```python
from build123d import *

# Parameters (mm, degrees)
SKETCH1_W           = 38.1
SKETCH1_H           = 38.1
SKETCH1_R           = 1.27
BOSS_EXTRUDE1_DEPTH = 6.35
CUT_EXTRUDE1_DEPTH  = 5.08
CUT_EXTRUDE2_REACH  = 29.679
SKETCH3_W           = 9.398
SKETCH3_H           = 21.59
SKETCH4_W           = 2.320401775
SKETCH4_H           = 5.08
SKETCH4_R           = 3.101894328
CUT_EXTRUDE3_DEPTH  = 28.679008291


with BuildPart() as part:
    # Sketch1 → Boss-Extrude1 (new body)
    with BuildSketch(Plane(origin=(0, 0, 0), x_dir=(1, 0, 0), z_dir=(0, 1, 0))):
        Rectangle(SKETCH1_W, SKETCH1_H)
        with Locations(Location((-17.018, 17.018, 0), (0, 0, 270))):
            Circle(SKETCH1_R, mode=Mode.SUBTRACT)
        with Locations(Location((-17.018, -17.018, 0), (0, 0, 90))):
            Circle(SKETCH1_R, mode=Mode.SUBTRACT)
        with Locations(Location((17.018, -17.018, 0), (0, 0, 270))):
            Circle(SKETCH1_R, mode=Mode.SUBTRACT)
        with Locations(Location((17.018, 17.018, 0), (0, 0, 90))):
            Circle(SKETCH1_R, mode=Mode.SUBTRACT)
    extrude(amount=BOSS_EXTRUDE1_DEPTH)

    # Sketch2 → Cut-Extrude1 (cut)
    with BuildSketch(Plane(origin=(0, 6.35, 0), x_dir=(1, 0, 0), z_dir=(0, 1, 0))):
        with BuildLine():
            Line((18.256262039, 13.97), (18.256262039, -13.97))
            ThreePointArc((18.256262039, -13.97), (15.324054183, -14.987286066), (13.97, -17.78))
            Line((13.97, -17.78), (-13.97, -17.78))
            ThreePointArc((-13.97, -17.78), (-15.324054183, -14.987286066), (-18.256262039, -13.97))
            Line((-18.256262039, -13.97), (-18.256262039, 13.97))
            ThreePointArc((-18.256262039, 13.97), (-15.324054183, 14.987286066), (-13.97, 17.78))
            Line((-13.97, 17.78), (13.97, 17.78))
            ThreePointArc((13.97, 17.78), (15.324054183, 14.987286066), (18.256262039, 13.97))
        make_face()
    extrude(amount=-CUT_EXTRUDE1_DEPTH, mode=Mode.SUBTRACT)

    # Sketch3 → Cut-Extrude2 (cut, up to next)
    with BuildSketch(Plane.XZ, mode=Mode.PRIVATE) as cut_extrude2_sk1:
        with Locations((-7.493, 0.635)):
            Rectangle(SKETCH3_W, SKETCH3_H)
    cut_extrude2_tool1 = extrude(cut_extrude2_sk1.sketch, amount=-CUT_EXTRUDE2_REACH, mode=Mode.PRIVATE) & part.part
    add(cut_extrude2_tool1.solids().sort_by_distance((-7.493, 0, 0.635))[0], mode=Mode.SUBTRACT)

    # Sketch4 → Cut-Extrude3 (cut, through all)
    with BuildSketch(Plane.XZ):
        with Locations((20.210200888, 0)):
            Rectangle(SKETCH4_W, SKETCH4_H)
        with Locations((17.889799113, 0)):
            Rectangle(SKETCH4_W, SKETCH4_H)
        with Locations(Location((2.54, 2.54, 0), (0, 0, 270))):
            Circle(SKETCH4_R)
    extrude(amount=-CUT_EXTRUDE3_DEPTH, mode=Mode.SUBTRACT)


solid = part.part
```
Read the model definition and answer for the solid it produces. Units are mm, in the model's axes. A direction names the side the tool comes from. Give positions to 0.01 mm unless a question says otherwise; leave off trailing zeros. Loops run counter-clockwise (first coordinate to the right, second up) from the corner with the lowest first, then second, coordinate; pieces in that order, holes last.
Item 1: For faces 5 (the flat face through (-8, 1, 11.43)), 6 (the flat face through (0, 4, 17.78)), 7 (the flat face through (16.73, 1, 0)), determine the directions among +Z, -Z, +X, -X, +Y, -Y from which every point of the face is accessible in a straight line to the end or side of a thin tool.
Item 2: The mould has two halves that part along X. Classify faces 1 (the cylindrical face through (-15.778, 3.131, 17.293)), 2 (the flat face through (19.05, 3, -11)), 3 (the flat face through (-12.192, 1, 0)), 4 (the flat face through (-18.43, 6.35, -1.5)): released by +X, released by -X, zero draft, split by the parting line, or undercut.
Item 3: The part is cut by section C-C (z = 3). Write down the section's boundary in (x, y), and give its area (3 significant figures).
Item 4: The part is cut by section B-B (z = 10). Write down the section's boundary in (x, y), and give its area (3 significant figures).
Item 5: Find the intervals of material crossed by line 1 along Z through (x, y) = (9, 3.25); line 2 along X through (y, z) = (2.25, -12.5); line 3 along Y through (x, z) = (1.5, -3), in increasing order.
Item 6: The part is cut by section A-A (x = -10). Write down the section's boundary in (y, z).
Item 7: This flat-tipped pin is pushed along its axis until it touches: pin 1 Ø3 at (x, z) = (3, -2) entering from +Y. Where does it stop, or does it pass through?
Item 8: The part is cut by section D-D (y = 2). Write down the section's boundary in (x, z), and give its area (3 significant figures).
Taken from the geometry:
1. face 5: +Y, -Y
1. face 6: +Y
1. face 7: +X, +Y, -Y
2. face 1: undercut
2. face 2: released by +X
2. face 3: undercut
2. face 4: zero draft
3. outline: (-19.05, 0) - (-12.19, 0) - (-12.19, 1.27) - (-18.26, 1.27) - (-18.26, 6.35) - (-19.05, 6.35) - close; (-2.79, 0) - (-0.53, 0) - (-0.53, 1.27) - (-2.79, 1.27) - close; (5.61, 0) - (19.05, 0) - (19.05, 6.35) - (18.26, 6.35) - (18.26, 1.27) - (5.61, 1.27) - close
3. area: 36.7 mm2
4. outline: (-19.05, 0) - (-12.19, 0) - (-12.19, 1.27) - (-18.26, 1.27) - (-18.26, 6.35) - (-19.05, 6.35) - close; (-2.79, 0) - (19.05, 0) - (19.05, 6.35) - (18.26, 6.35) - (18.26, 1.27) - (-2.79, 1.27) - close
4. area: 44.5 mm2
5. line 1: z = -19.05 to -17.78, 17.78 to 19.05
5. line 2: x = -19.05 to -18.26, 18.26 to 19.05
5. line 3: y = 0 to 1.27
6. outline: (0, -19.05) - (6.35, -19.05) - (6.35, -17.78) - (1.27, -17.78) - (1.27, -10.16) - (0, -10.16) - close; (0, 11.43) - (1.27, 11.43) - (1.27, 17.78) - (6.35, 17.78) - (6.35, 19.05) - (0, 19.05) - close
7. pin 1: stops at y = 1.27
8. outline: (-19.05, -19.05) - (19.05, -19.05) - (19.05, -2.54) - (18.26, -2.54) - (18.26, -13.97) arc R4.06 ccw to (13.97, -17.78) - (-13.97, -17.78) arc R4.06 ccw to (-18.26, -13.97) - (-18.26, 13.97) arc R4.06 ccw to (-13.97, 17.78) - (13.97, 17.78) arc R4.06 ccw to (18.26, 13.97) - (18.26, 2.54) - (19.05, 2.54) - (19.05, 19.05) - (-19.05, 19.05) - close; hole circle Ø2.54 at (-17.02, -17.02); hole circle Ø2.54 at (-17.02, 17.02); hole circle Ø2.54 at (17.02, -17.02); hole circle Ø2.54 at (17.02, 17.02)
8. area: 180 mm2
